Work out the finished part from the listing and answer in its coordinate system (mm). A direction names the side the tool comes from. Coordinates: 2 decimals unless noted, no trailing zeros. Loops run counter-clockwise (first coordinate to the right, second up) from the corner with the lowest first, then second, coordinate; pieces in that order, holes last. Notation, with made-up numbers: M -21,59 L 36,59 A23 ccw 36,67 Z; hole C 77,17.25 d11. An arc over 180 degrees is marked long. Write each question's results on one line, items separated by ' | '.
```python
from build123d import *

# Parameters (mm, degrees)
SKETCH1_W           = 203.2
SKETCH1_H           = 203.2
SKETCH1_W_2         = 190.5
SKETCH1_H_2         = 190.5
BOSS_EXTRUDE1_DEPTH = 1.27
SKETCH2_W           = 6.35
SKETCH2_H           = 190.5
BOSS_EXTRUDE2_DEPTH = 1.27
CUT_EXTRUDE1_DEPTH  = 1.27


with BuildPart() as part:
    # Sketch1 → Boss-Extrude1 (new body, symmetric)
    with BuildSketch(Plane(origin=(0, 0, 0), x_dir=(1, 0, 0), z_dir=(0, 1, 0))):
        Rectangle(SKETCH1_W, SKETCH1_H)
        Rectangle(SKETCH1_W_2, SKETCH1_H_2, mode=Mode.SUBTRACT)
    extrude(amount=BOSS_EXTRUDE1_DEPTH, both=True)

    # Sketch2 → Boss-Extrude2 (add, symmetric)
    with BuildSketch(Plane(origin=(0, 0, 0), x_dir=(1, 0, 0), z_dir=(0, 1, 0))):
        with Locations((92.075, 0)):
            Rectangle(SKETCH2_W, SKETCH2_H)
    extrude(amount=BOSS_EXTRUDE2_DEPTH, both=True)

    # Sketch3 → Cut-Extrude1 (cut)
    with BuildSketch(Plane(origin=(0, 1.27, 0), x_dir=(1, 0, 0), z_dir=(0, 1, 0))):
        Polygon((101.6, 40.64), (95.25, 34.29), (95.25, 67.31), (101.6, 60.96), align=None)
        Polygon((101.6, -60.96), (101.6, -40.64), (95.25, -34.29), (95.25, -67.31), align=None)
    extrude(amount=-CUT_EXTRUDE1_DEPTH, mode=Mode.SUBTRACT)


solid = part.part
```
1) Straight lines are drawn through the part: probe 1 along X at (y, z) = (-1.1, 72.5); probe 2 along Z at (x, y) = (51.5, 0.4); probe 3 along X at (y, z) = (0.7, 48). For each, find the intervals that lie inside material, in ascending order. Write a range as [from, to].
Check result:
probe 1: [-101.6, -95.25], [88.9, 101.6] | probe 2: [-101.6, -95.25], [95.25, 101.6] | probe 3: [-101.6, -95.25], [88.9, 95.25]
2) Find section B-B, the plane x = -56. Give the vertices of the cut face in (y, z).
Check result:
outline: M -1.27,-101.6 L 1.27,-101.6 L 1.27,-95.25 L -1.27,-95.25 Z; M -1.27,95.25 L 1.27,95.25 L 1.27,101.6 L -1.27,101.6 Z
3) Given pin 1 Ø0.6 at (y, z) = (0.5, 58) entering from +X; pin 2 Ø5 at (x, z) = (98.5, -56.5) entering from +Y, each flat-ended and moving along its own axis, determine where each tip first touches the part or whether it passes through.
Check result:
pin 1: x = 95.25 | pin 2: y = 0
4) Find section D-D, the plane z = 49. Give the vertices of the cut face in (x, y), and give its area (3 significant figures).
Check result:
outline: M -101.6,-1.27 L -95.25,-1.27 L -95.25,1.27 L -101.6,1.27 Z; M 88.9,-1.27 L 101.6,-1.27 L 101.6,0 L 95.25,0 L 95.25,1.27 L 88.9,1.27 Z | area: 40.3 mm^2
5) Find section A-A, the plane z = -24.5. Give the vertices of the cut face in (x, y), and give its area (3 significant figures).
Check result:
outline: M -101.6,-1.27 L -95.25,-1.27 L -95.25,1.27 L -101.6,1.27 Z; M 88.9,-1.27 L 101.6,-1.27 L 101.6,1.27 L 88.9,1.27 Z | area: 48.4 mm^2
6) Which of the six approach directions +Z, -Z, +X, -X, +Y, -Y give full straight-line access (tool end or side, diameter ignored) to faces 1 (the face through (98, 0, 51)), 2 (the face through (90, 1.27, 7))?
Check result:
face 1: +Y | face 2: +Z, -Z, +X, -X, +Y
7) For a pull along Z with two mould halves and no side action, classify faces 3 (the face through (98.47, 0.64, 37.51)), 4 (the face through (90, -1.27, 7)), 5 (the face through (98, 0, -51)) as released by +Z, released by -Z, zero draft, split by the parting line, or undercut.
Check result:
face 3: undercut | face 4: zero draft | face 5: undercut
8) Find section C-C, the plane y = -0.45. Give the vertices of the cut face in (x, z).
Check result:
outline: M -101.6,-101.6 L 101.6,-101.6 L 101.6,101.6 L -101.6,101.6 Z; hole M -95.25,-95.25 L 88.9,-95.25 L 88.9,95.25 L -95.25,95.25 Z
